Verification items for the finished model (mm, model axes). A direction names the side the tool comes from. Round coordinates to 2 decimals unless told otherwise and drop trailing zeros. Order: outer loops, then holes, each group sorted by start corner. A loop starts at its lowest first (then second) coordinate and runs counter-clockwise, first axis right, second up. Notation, with made-up numbers: M 65.5,63.25 L 81.5,63.25 A30 cw 81.5,94.25 Z; hole C 46,64.25 d1. An arc over 180 degrees is marked long. Use one line per item in the form item = value. Start each with the question number.
Item 1: Cross-section at B-B on x = 0. Enter the section's corners in (y, z).
Item 2: Cross-section at A-A on z = 3.75. Enter the section's corners in (x, y), then the cut area to 3 significant figures.
Item 3: Cross-section at D-D on x = -7.25. Enter the section's corners in (y, z), then the cut area to 3 significant figures.
Item 4: Release check for a two-part mould opening along X. For faces 1 (the flat face through (-4, -3, 7)), 2 (the flat face through (-5, 4, 4)), 3 (the cylindrical face through (0, 4, 7)), 4 (the cylindrical face through (0, -4, 7)) record: +X half, -X half, draft (parallel to the pull), parting line (faces both ways), or undercut.
Item 5: Tool access check on faces 5 (the flat face through (-0.1, 4.2, 8)), 6 (the flat face through (-7, -3, 3)), 7 (the flat face through (4, 3, 7)). Record the directions out of +Z, -Z, +X, -X, +Y, -Y that give a thin tool (end or side, any length) a straight path to the whole face; none if there is none.
Item 6: Thickness scan on probe 1 along X at (y, z) = (0, 2.75); probe 2 along Y at (x, z) = (0, 1.25); probe 3 along X at (y, z) = (1.5, 3). Record the ranges inside material, lowest first. Write a range as [from, to].
Item 7: Go/stop test with flat-tipped pins: pin 1 Ø4 at (x, y) = (-3.5, 0) entering from -Z; pin 2 Ø1 at (y, z) = (4.5, 5.5) entering from -X; pin 3 Ø1 at (x, z) = (-7, 2) entering from -Y. Record where each tip stops, or that it passes through.
Item 8: Cross-section at C-C on x = 4.25. Enter the section's corners in (y, z), then the cut area to 3 significant figures.
from build123d import *

# Parameters (mm, degrees)
SKETCH1_R           = 2
BOSS_EXTRUDE1_DEPTH = 8
SKETCH2_W           = 2
SKETCH2_H           = 6
CUT_EXTRUDE1_DEPTH  = 18
SKETCH3_R           = 4
CUT_EXTRUDE2_DEPTH  = 36


with BuildPart() as part:
    # Sketch1 → Boss-Extrude1 (new body)
    with BuildSketch(Plane.XY):
        with BuildLine():
            Line((-5, 3), (-8.235644223, 3))
            ThreePointArc((-8.235644223, 3), (-10.359234513, 2.119047966), (-11.235637346, -0.006423812))
            ThreePointArc((-11.235637346, -0.006423812), (-10.354692189, -2.12359029), (-8.235644223, -3))
            Line((-8.235644223, -3), (-5, -3))
            Line((-5, -3), (-5, -5))
            Line((-5, -5), (5, -5))
            Line((5, -5), (5, 5))
            Line((5, 5), (-5, 5))
            Line((-5, 5), (-5, 3))
        make_face()
        with Locations((-8.235644223, 0)):
            Circle(SKETCH1_R, mode=Mode.SUBTRACT)
        Circle(SKETCH1_R, mode=Mode.SUBTRACT)
    extrude(amount=BOSS_EXTRUDE1_DEPTH)

    # Sketch2 → Cut-Extrude1 (cut, symmetric)
    with BuildSketch(Plane(origin=(0, 0, 0), x_dir=(0, 0, -1), z_dir=(1, 0, 0))):
        with Locations((-7, 0)):
            Rectangle(SKETCH2_W, SKETCH2_H)
    extrude(amount=CUT_EXTRUDE1_DEPTH, both=True, mode=Mode.SUBTRACT)

    # Sketch3 → Cut-Extrude2 (cut)
    with BuildSketch(Plane.XY.offset(6)):
        Circle(SKETCH3_R)
    extrude(amount=CUT_EXTRUDE2_DEPTH, mode=Mode.SUBTRACT)


solid = part.part
Output values:
q1.outline = M -5,0 L -2,0 L -2,6 L -4,6 L -4,8 L -5,8 Z; M 2,0 L 5,0 L 5,8 L 4,8 L 4,6 L 2,6 Z
q2.outline = M -8.24,-3 L -5,-3 L -5,-5 L 5,-5 L 5,5 L -5,5 L -5,3 L -8.24,3 A3 ccw Z; hole C -8.24,0 d4; hole C 0,0 d4
q2.area = 108 mm2
q3.outline = M -3,0 L -1.74,0 L -1.74,6 L -3,6 Z; M 1.74,0 L 3,0 L 3,6 L 1.74,6 Z
q3.area = 15.1 mm2
q4.face_1 = draft
q4.face_2 = -X half
q4.face_3 = undercut
q4.face_4 = undercut
q5.face_5 = +Z, +X, -X, +Y, -Y
q5.face_6 = +Z, -Z, -X, -Y
q5.face_7 = +Z, +X, -X
q6.probe_1 = [-11.24, -10.24], [-6.24, -2], [2, 5]
q6.probe_2 = [-5, -2], [2, 5]
q6.probe_3 = [-10.83, -9.56], [-6.91, -1.32], [1.32, 5]
q7.pin_1 = 0
q7.pin_2 = -5
q7.pin_3 = -3
q8.outline = M -5,0 L 5,0 L 5,8 L 3,8 L 3,6 L -3,6 L -3,8 L -5,8 Z
q8.area = 68.0 mm2
